```python
from build123d import *

# Parameters (mm, degrees)
SKETCH1_W           = 25.4
SKETCH1_H           = 76.2
SKETCH1_W_2         = 4
BOSS_EXTRUDE1_DEPTH = 4
SKETCH1_3_W         = 4
SKETCH1_3_H         = 76.2
BOSS_EXTRUDE2_DEPTH = 10
FILLET1_R           = 1
CHAMFER1_SIZE       = 0.5


with BuildPart() as part:
    # Sketch1 → Boss-Extrude1 (new body)
    with BuildSketch(Plane.XY):
        with Locations((0, 12.7)):
            Rectangle(SKETCH1_W, SKETCH1_H)
        with Locations((14.7, 12.7)):
            Rectangle(SKETCH1_W_2, SKETCH1_H)
        with Locations((-14.7, 12.7)):
            Rectangle(SKETCH1_W_2, SKETCH1_H)
    extrude(amount=BOSS_EXTRUDE1_DEPTH)

    # Sketch1_3 → Boss-Extrude2 (add)
    with BuildSketch(Plane.XY):
        with Locations((-14.7, 12.7)):
            Rectangle(SKETCH1_3_W, SKETCH1_3_H)
        with Locations((14.7, 12.7)):
            Rectangle(SKETCH1_3_W, SKETCH1_3_H)
    extrude(amount=-BOSS_EXTRUDE2_DEPTH)

    # Fillet1
    fillet1_edges = [part.edges().sort_by_distance(p)[0] for p in [
        (16.7, -25.4, -3),
        (-12.7, 50.8, -5),
        (-12.7, -25.4, -5),
        (12.7, -25.4, -5),
        (12.7, 50.8, -5),
        (-16.7, -25.4, -3),
        (-16.7, 50.8, -3),
        (16.7, 50.8, -3),
    ]]
    fillet(fillet1_edges, radius=FILLET1_R)

    # Chamfer1
    chamfer1_edges = [part.edges().sort_by_distance(p)[0] for p in [
        (0, -25.4, 0),
        (0, 50.8, 0),
        (-14.7, 50.8, -10),
        (0, 50.8, 4),
        (14.7, 50.8, -10),
        (12.7, 12.7, -10),
        (16.7, 12.7, -10),
        (14.7, -25.4, -10),
        (16.407106781, 50.507106781, -10),
        (16.407106781, -25.107106781, -10),
        (12.992893219, -25.107106781, -10),
        (12.992893219, 50.507106781, -10),
        (-12.7, 12.7, -10),
        (-14.7, -25.4, -10),
        (-16.7, 12.7, -10),
        (-16.407106781, 50.507106781, -10),
        (-16.407106781, -25.107106781, -10),
        (-12.992893219, -25.107106781, -10),
        (-12.992893219, 50.507106781, -10),
        (0, -25.4, 4),
        (-16.7, 12.7, 4),
        (16.7, 12.7, 4),
        (-16.407106781, 50.507106781, 4),
        (16.407106781, 50.507106781, 4),
        (16.407106781, -25.107106781, 4),
        (-16.407106781, -25.107106781, 4),
    ]]
    chamfer(chamfer1_edges, length=CHAMFER1_SIZE)


solid = part.part
```
Model file for the job. Use its own axes, mm. A direction names the side the tool comes from. Coordinates: 2 decimals unless noted, no trailing zeros. Order: outer loops, then holes, each group sorted by start corner. A loop starts at its lowest first (then second) coordinate and runs counter-clockwise, first axis right, second up. Notation, with made-up numbers: M 12,34 L 42,34 A16 cw 42,59 Z; hole C 56,-37 d7. An arc over 180 degrees is marked long. Answer as CSV lines item,"result".
(1) Band-saw the part on C-C, the plane y = -17. List the corners of the cut face in (x, z), then the cut area to 3 significant figures.
Geometry says:
outline,"M -16.7,-9.5 L -16.2,-10 L -13.2,-10 L -12.7,-9.5 L -12.7,0 L 12.7,0 L 12.7,-9.5 L 13.2,-10 L 16.2,-10 L 16.7,-9.5 L 16.7,3.5 L 16.2,4 L -16.2,4 L -16.7,3.5 Z"
area,"213 mm2"
(2) Band-saw the part on B-B, the plane x = 7. List the corners of the cut face in (y, z), then the cut area to 3 significant figures.
Geometry says:
outline,"M -25.4,0.5 L -24.9,0 L 50.3,0 L 50.8,0.5 L 50.8,3.5 L 50.3,4 L -24.9,4 L -25.4,3.5 Z"
area,"304 mm2"
(3) Band-saw the part on A-A, the plane z = -1. List the corners of the cut face in (x, y), then the cut area to 3 significant figures.
Geometry says:
outline,"M -16.7,-24.4 A1 ccw -15.7,-25.4 L -13.7,-25.4 A1 ccw -12.7,-24.4 L -12.7,49.8 A1 ccw -13.7,50.8 L -15.7,50.8 A1 ccw -16.7,49.8 Z; M 12.7,-24.4 A1 ccw 13.7,-25.4 L 15.7,-25.4 A1 ccw 16.7,-24.4 L 16.7,49.8 A1 ccw 15.7,50.8 L 13.7,50.8 A1 ccw 12.7,49.8 Z"
area,"608 mm2"
(4) Pull direction X, two halves, no side cores. Call faces 1 (the flat face through (0, 13, 0)), 2 (the flat face through (16.7, 12, -3)), 3 (the flat face through (0, -25.4, 1)): +X half, -X half, draft (parallel to the pull), parting line (faces both ways), or undercut.
Geometry says:
face 1,"undercut"
face 2,"+X half"
face 3,"draft"
(5) Wall check: line 1 along X through (y, z) = (2.5, -2.5); line 2 along Z through (x, y) = (-8, 21); line 3 along Y through (x, z) = (-13, -0.5). Give the ranges that are in metal, low to high.
Geometry says:
line 1,"x = -16.7 to -12.7, 12.7 to 16.7"
line 2,"z = 0 to 4"
line 3,"y = -25.11 to 50.51"
(6) 3-axis set-ups, long thin cutter, end or side, ignore diameter. For faces 4 (the flat face through (0, 13, 4)), 5 (the flat face through (-12.7, 12, -5)): which of +Z, -Z, +X, -X, +Y, -Y reach the whole face in a straight line?
Geometry says:
face 4,"+Z, +X, -X, +Y, -Y"
face 5,"-Z, +Y, -Y"
(7) Flat gauge pin, fed straight in: pin 1 (4 mm diameter, centred on x = -7.5, z = 0, fed in from -Y). Where does the tip first touch, or does it go through?
Geometry says:
pin 1,"stops at y = -25.4"
